Geometry: final body of the model. Coordinates: model frame, mm. Round coordinates to 2 decimals unless told otherwise and drop trailing zeros. Write each loop counter-clockwise with the first axis right and the second up, starting at its lowest first coordinate (ties: lowest second). Pieces come first, ordered by that corner, then holes. Notation, with made-up numbers: M 52,65.25 L 75,65.25 A23 ccw 75,84.25 Z; hole C -28,23 d3. An arc over 180 degrees is marked long. Use one line per item in the form item = value. Start each with the question number.
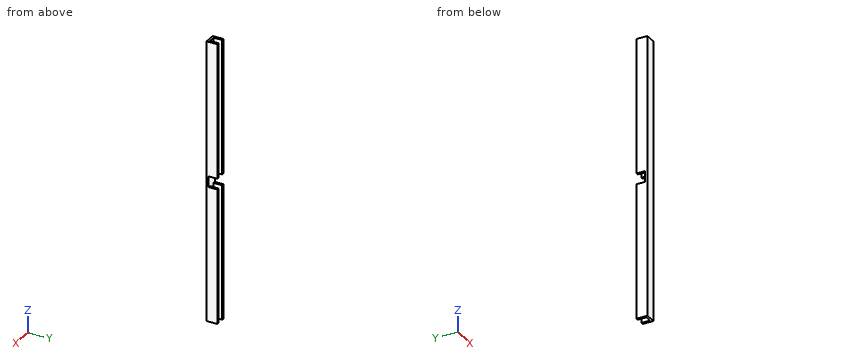
from build123d import *

# Parameters (mm, degrees)
BOSS_EXTRU_1_DEPTH      = 260
ENL_V_MAT_EXTRU_1_DEPTH = 8


with BuildPart() as part:
    # Esquisse1 → Boss.-Extru.1 (new body)
    with BuildSketch(Plane.XY):
        Polygon((0, 0), (0, -10), (10, -10), (10, 0), (8, 0), (8, -8), (2, -8), (2, 0), align=None)
    extrude(amount=BOSS_EXTRU_1_DEPTH)

    # Esquisse2 → Enlèv. mat.-Extru.1 (cut)
    with BuildSketch(Plane(origin=(0, 0, 0), x_dir=(1, 0, 0), z_dir=(0, 1, 0))):
        Polygon((-8.996226047, -125), (31.208128552, -125), (31.208128552, -127.984639705), (31.208128552, -135), (-8.996226047, -135), align=None)
    extrude(amount=-ENL_V_MAT_EXTRU_1_DEPTH, mode=Mode.SUBTRACT)


solid = part.part
1. Section query B-B (z = 238). Return loops of the section in (x, y), then the cut area to 3 significant figures.
2. Ray query, probe 1 along X at (y, z) = (-7, 240.5); probe 2 along Z at (x, y) = (1.75, -6); probe 3 along Y at (x, z) = (5.5, 150). Return the intervals inside material, ascending.
3. Section query A-A (y = -4.75). Return loops of the section in (x, z).
4. Section query C-C (z = 132.5). Return loops of the section in (x, y).
5. Contact query for a flat-ended pin moving along its axis: pin 1 (1.6 mm diameter, centred on x = 9, y = -5.5, fed in from -Z). Output: stop coordinate, or through.
Checks:
q1.outline = M 0,-10 L 10,-10 L 10,0 L 8,0 L 8,-8 L 2,-8 L 2,0 L 0,0 Z
q1.area = 52.0 mm^2
q2.probe_1 = 0 to 2, 8 to 10
q2.probe_2 = 0 to 125, 135 to 260
q2.probe_3 = -10 to -8
q3.outline = M 0,0 L 2,0 L 2,125 L 0,125 Z; M 0,135 L 2,135 L 2,260 L 0,260 Z; M 8,0 L 10,0 L 10,125 L 8,125 Z; M 8,135 L 10,135 L 10,260 L 8,260 Z
q4.outline = M 0,-10 L 10,-10 L 10,-8 L 0,-8 Z
q5.pin_1 = 0
